from build123d import *

# Parameters (mm, degrees)
PAD001_DEPTH = 6
SKETCH_R     = 7.5
PAD_DEPTH    = 26
SKETCH003_W  = 17.6
SKETCH003_H  = 1.5
POCKET_DEPTH = 6
SKETCH004_R  = 3.3
HOLE_DEPTH   = 18
HOLE_TIPS_R  = 3.3


with BuildPart() as body001:
    # Sketch002 → Pad001 (new body)
    with BuildSketch(Plane.XY.offset(5)):
        Polygon((6, 3.464102), (6, -26.535898), (-6, -26.535898), (-6, 3.464102), (0, 6.928203), align=None)
    extrude(amount=PAD001_DEPTH)


with BuildPart() as body:
    # Sketch → Pad (new body)
    with BuildSketch(Plane.XY):
        Circle(SKETCH_R)
    extrude(amount=PAD_DEPTH)

    # Boolean: cut Body001
    add(body001.part, mode=Mode.SUBTRACT)

    # Sketch003 (on Face3 of Boolean) → Pocket (cut)
    with BuildSketch(Plane.XY.offset(26)):
        Rectangle(SKETCH003_W, SKETCH003_H)
    extrude(amount=-POCKET_DEPTH, mode=Mode.SUBTRACT)

    # Sketch004 (on Face7 of Pocket) → Hole (cut)
    with BuildSketch(Plane(origin=(0, 0, 0), x_dir=(1, 0, 0), z_dir=(0, 0, -1))):
        Circle(SKETCH004_R)
    extrude(amount=-HOLE_DEPTH, mode=Mode.SUBTRACT)

    # Hole tips → Hole tip 1 section 0
    with BuildSketch(Plane(origin=(0, 0, 18), x_dir=(1, 0, 0), z_dir=(0, 0, -1)), mode=Mode.PRIVATE) as hole_tip_1_s0:
        Circle(HOLE_TIPS_R)
    loft([hole_tip_1_s0.sketch, Vertex(0, 0, 19.98284)], mode=Mode.SUBTRACT)


solid = body.part
Geometry check sheet. Reference: the model listing, model coordinates, mm. A direction names the side the tool comes from. Give positions to 0.01 mm unless a question says otherwise; leave off trailing zeros. Order: outer loops, then holes, each group sorted by start corner. A loop starts at its lowest first (then second) coordinate and runs counter-clockwise, first axis right, second up. Notation, with made-up numbers: (10.5, -7.5) - (24.5, -7.5) arc R18 ccw to (24.5, -2.5) - close; hole circle Ø3 at (46.25, 15.5). An arc over 180 degrees is marked (long way). Answer as a JSON object with one key per item and string values.
(1) Cross-section at A-A (y = 4). Record the cut outline in (x, z), then the cut area to 3 significant figures.
Report:
{"outline": "(-6.34, 0) - (6.34, 0) - (6.34, 26) - (-6.34, 26) - close; hole (-5.07, 5) - (5.07, 5) - (5.07, 11) - (-5.07, 11) - close", "area": "269 mm^2"}
(2) Cross-section at B-B (y = -5.5). Record the cut outline in (x, z).
Report:
{"outline": "(-5.1, 0) - (5.1, 0) - (5.1, 5) - (-5.1, 5) - close; (-5.1, 11) - (5.1, 11) - (5.1, 26) - (-5.1, 26) - close"}
(3) Tool access check on faces 4 (the cylindrical face through (-2.43, -2.23, 2.46)), 5 (the flat face through (6, 0, 8)), 6 (the flat face through (0, -0.75, 23)), 7 (the flat face through (0, 3, 26)), 8 (the cylindrical face through (4.032, 6.324, 12.818)). Record the directions out of +Z, -Z, +X, -X, +Y, -Y that give a thin tool (end or side, any length) a straight path to the whole face; none if there is none.
Report:
{"face 4": "-Z", "face 5": "-Y", "face 6": "+Z, +X, -X", "face 7": "+Z, +X, -X, +Y, -Y", "face 8": "+Z, -Z"}
(4) Cross-section at C-C (z = 12). Record the cut outline in (x, y), then the cut area to 3 significant figures.
Report:
{"outline": "circle Ø15 at (0, 0); hole circle Ø6.6 at (0, 0)", "area": "143 mm^2"}
(5) Draft check along Z on faces 1 (the flat face through (-0.1, 0.3, 20)), 2 (the flat face through (-1.2, -3.4, 11)), 3 (the cylindrical face through (-2.43, -2.23, 14.45)). Enter one of: released by +Z, released by -Z, zero draft, split by the parting line, or undercut.
Report:
{"face 1": "released by +Z", "face 2": "undercut", "face 3": "zero draft"}
(6) Cross-section at D-D (x = 6.5). Record the cut outline in (y, z), then the cut area to 3 significant figures.
Report:
{"outline": "(-3.74, 0) - (3.74, 0) - (3.74, 26) - (0.75, 26) - (0.75, 20) - (-0.75, 20) - (-0.75, 26) - (-3.74, 26) - close", "area": "186 mm^2"}
(7) Material ranges on line 1 (X direction, y = 0, z = 2.8); line 2 (Z direction, x = 1.25, y = -4.5), recorded low to high.
Report:
{"line 1": "-7.5 to -3.3, 3.3 to 7.5", "line 2": "0 to 5, 11 to 26"}
(8) Depth check by flat-ended pin: pin 1 Ø1.2 at (x, y) = (-1, 0) entering from +Z; pin 2 Ø3 at (y, z) = (-3, 12) entering from +X; pin 3 Ø4 at (y, z) = (-4, 20.5) entering from -X. Enter the tip coordinate at first touch or a pass-through.
Report:
{"pin 1": "z = 20", "pin 2": "x = 7.35", "pin 3": "x = -7.23"}
